Geometry check sheet. Reference: the model listing, model coordinates, mm. Face numbers are marked on the shaded views. A direction names the side the tool comes from. Give positions to 0.01 mm unless a question says otherwise; leave off trailing zeros. Write each loop counter-clockwise with the first axis right and the second up, starting at its lowest first coordinate (ties: lowest second). Pieces come first, ordered by that corner, then holes. Notation, with made-up numbers: (-38, 18.5) -> (12, 18.5) arc R12 ccw to (12, 35.5) -> close; hole circle Ø2 at (79, -12.75). An arc over 180 degrees is marked (long way). Write item = value, one per line. Start each with the question number.
1. Thickness scan on line 1 along Y through (x, z) = (7, -6.4); line 2 along Y through (x, z) = (8, -4); line 3 along Z through (x, y) = (9.75, 26.5). Record the ranges inside material, lowest first.
2. Set-up check for the marked faces 1, 2, 3, 4 and 5: record each of +Z, -Z, +X, -X, +Y, -Y from which the full face is reachable in a straight line by a thin tool's end or side.
3. Cross-section at A-A, the plane z = -5.75. Record the cut outline in (x, y).
4. Mould release check, pull along Y, two halves, no side actions. Record for the marked faces 6, 7 and 8: pulls with the +Y half, pulls with the -Y half, needs draft (parallel to the pull), parting line crosses it, or undercut.
5. Depth check by flat-ended pin: P1, Ø1.5, axis at y = 11, z = 1.5, coming from the +X side; P2, Ø5, axis at x = 5.5, y = -8.5, coming from the +Z side; P3, Ø2, axis at x = 13.5, z = -3.5, coming from the +Y side. Enter the tip coordinate at first touch or a pass-through.
6. Cross-section at C-C, the plane y = -9. Record the cut outline in (x, z).
7. Cross-section at D-D, the plane z = -0.5. Record the cut outline in (x, y).
8. Cross-section at B-B, the plane x = 7. Record the cut outline in (y, z), plus the area to 3 significant figures.
```python
from build123d import *

# Parameters (mm, degrees)
SKETCH_W     = 14
SKETCH_H     = 22
PAD_DEPTH    = 3
SKETCH001_W  = 14
SKETCH001_H  = 3
PAD001_DEPTH = 7.6
SKETCH002_W  = 17
SKETCH002_H  = 17
SKETCH002_R  = 2.5
PAD002_DEPTH = 3
FILLET_R     = 2
FILLET001_R  = 1


with BuildPart() as part:
    # Sketch → Pad (new body)
    with BuildSketch(Plane.XY):
        with Locations((7, 11)):
            Rectangle(SKETCH_W, SKETCH_H)
    extrude(amount=PAD_DEPTH)

    # Sketch001 → Pad001 (join)
    with BuildSketch(Plane.XY):
        with Locations((7, 20.5)):
            Rectangle(SKETCH001_W, SKETCH001_H)
        with Locations((7, 1.5)):
            Rectangle(SKETCH001_W, SKETCH001_H)
    extrude(amount=-PAD001_DEPTH)

    # Sketch002 → Pad002 (join)
    with BuildSketch(Plane.XY.offset(-4.6)):
        with Locations((8.5, 30.5)):
            Rectangle(SKETCH002_W, SKETCH002_H)
        with Locations((7, 31)):
            Circle(SKETCH002_R, mode=Mode.SUBTRACT)
        with Locations((8.5, -8.5)):
            Rectangle(SKETCH002_W, SKETCH002_H)
        with Locations((7, -9)):
            Circle(SKETCH002_R, mode=Mode.SUBTRACT)
    extrude(amount=-PAD002_DEPTH)

    # Fillet
    fillet_edges = [part.edges().sort_by_distance(p)[0] for p in [
        (17, -17, -6.1),
        (17, 0, -6.1),
        (17, 22, -6.1),
        (17, 39, -6.1),
    ]]
    fillet(fillet_edges, radius=FILLET_R)

    # Fillet001
    fillet001_edges = [part.edges().sort_by_distance(p)[0] for p in [
        (0, -17, -6.1),
        (0, 39, -6.1),
    ]]
    fillet(fillet001_edges, radius=FILLET001_R)


solid = part.part
```
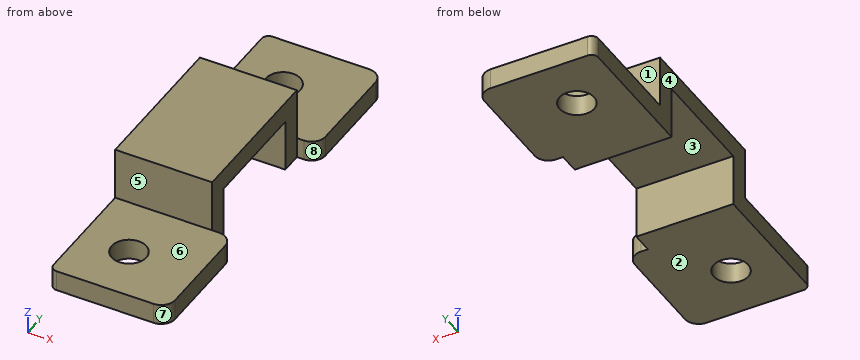
Answers:
q1.line_1 = -17 to -11.5, -6.5 to 3, 19 to 28.5, 33.5 to 39
q1.line_2 = 0 to 3, 19 to 22
q1.line_3 = -7.6 to -4.6
q2.face_1 = +Z, +X, -X, +Y
q2.face_2 = -Z, +X, -X, +Y, -Y
q2.face_3 = -Z, +X, -X
q2.face_4 = +Z, -Z, -X, +Y, -Y
q2.face_5 = +Z, +X, -X, -Y
q3.outline = (0, -16) arc R1 ccw to (1, -17) -> (15, -17) arc R2 ccw to (17, -15) -> (17, -2) arc R2 ccw to (15, 0) -> (14, 0) -> (14, 3) -> (0, 3) -> close; (0, 19) -> (14, 19) -> (14, 22) -> (15, 22) arc R2 ccw to (17, 24) -> (17, 37) arc R2 ccw to (15, 39) -> (1, 39) arc R1 ccw to (0, 38) -> close; hole circle Ø5 at (7, -9); hole circle Ø5 at (7, 31)
q4.face_6 = needs draft
q4.face_7 = pulls with the -Y half
q4.face_8 = undercut
q5.P1 = 14
q5.P2 = -4.6
q5.P3 = 22
q6.outline = (0, -7.6) -> (4.5, -7.6) -> (4.5, -4.6) -> (0, -4.6) -> close; (9.5, -7.6) -> (17, -7.6) -> (17, -4.6) -> (9.5, -4.6) -> close
q7.outline = (0, 0) -> (14, 0) -> (14, 3) -> (0, 3) -> close; (0, 19) -> (14, 19) -> (14, 22) -> (0, 22) -> close
q8.outline = (-17, -7.6) -> (-11.5, -7.6) -> (-11.5, -4.6) -> (-17, -4.6) -> close; (-6.5, -7.6) -> (3, -7.6) -> (3, 0) -> (19, 0) -> (19, -7.6) -> (28.5, -7.6) -> (28.5, -4.6) -> (22, -4.6) -> (22, 3) -> (0, 3) -> (0, -4.6) -> (-6.5, -4.6) -> close; (33.5, -7.6) -> (39, -7.6) -> (39, -4.6) -> (33.5, -4.6) -> close
q8.area = 184 mm^2
